Could you check a few things on this model? Use its own coordinates, in mm. A direction names the side the tool comes from. Coordinates: 2 decimals unless noted, no trailing zeros. Order: outer loops, then holes, each group sorted by start corner. A loop starts at its lowest first (then second) coordinate and runs counter-clockwise, first axis right, second up. Notation, with made-up numbers: (72.5, -29) - (123.5, -29) arc R31 cw to (123.5, 6) - close; hole circle Ø2 at (5.5, 34.25). An arc over 180 degrees is marked (long way). Answer as a JSON object with one key per item and string values. Group by question number.
(1) Which directions (+Z, -Z, +X, -X, +Y, -Y) give clear straight access to the entire face, cutting with the end or side of a thin tool? Please do faces 1 (the flat face through (0, -30.5, 2)), 2 (the flat face through (-85, 26, 2)), 3 (the flat face through (1.5, 42, 2)), 4 (the flat face through (-1.5, -42, 2)).
(2) We'd pull the mould along Y, two halves only. Please class faces 5 (the flat face through (-10, 46, 2)), 6 (the flat face through (6, 44.32, 2)), 7 (the flat face through (-85, -26, 2)): pulls with the +Y half, pulls with the -Y half, needs draft (parallel to the pull), parting line crosses it, or undercut.
(3) Please list where these lines run through material, in increasing order: probe 1 along Y at (x, z) = (38.5, 1.35); probe 2 along X at (y, z) = (-42, 1.85); probe 3 along X at (y, z) = (-6, 1.1).
(4) Imagine slicing it at C-C, the plane z = 0.9. Give the number of separate pieces and of enclosed holes in the cut face, and give its area (3 significant figures).
(5) Imagine slicing it at B-B, the plane y = 28.5. Write out the boundary of the cut face in (x, z).
(6) Will these pins go through, and if not, where does the flat tip stop? P1, Ø1.6, axis at y = -46, z = 1, coming from the +X side; P2, Ø1, axis at x = -2.5, z = 1.5, coming from the +Y side; P3, Ø0.6, axis at x = 2.5, z = 1.5, coming from the -Y side.
(7) Imagine slicing it at A-A, the plane x = -17.5. Write out the boundary of the cut face in (y, z), and give its area (3 significant figures).
from build123d import *

# Parameters (mm, degrees)
SKETCH1_W               = 180
SKETCH1_H               = 95
BOSS_EXTRUDE1_DEPTH     = 3.18
CUT_EXTRUDE1_START      = -4.18
SKETCH2_W               = 3.18
SKETCH2_H               = 37.625
CUT_EXTRUDE1_DEPTH      = 5.18
SKETCH3_R               = 1.55
CUT_EXTRUDE2_DEPTH      = 1
CUT_EXTRUDE2_DEPTH_BACK = 4.18
CUT_EXTRUDE3_START      = -4.18
CUT_EXTRUDE3_DEPTH      = 5.18
SKETCH7_W               = 98.6
SKETCH7_H               = 61.9
CUT_EXTRUDE6_DEPTH      = 1
CUT_EXTRUDE6_DEPTH_BACK = 4.18
SKETCH8_W               = 9
SKETCH8_H               = 52
CUT_EXTRUDE7_DEPTH      = 1
CUT_EXTRUDE7_DEPTH_BACK = 4.18


with BuildPart() as part:
    # Sketch1 → Boss-Extrude1 (new body)
    with BuildSketch(Plane.XY):
        Rectangle(SKETCH1_W, SKETCH1_H)
    extrude(amount=BOSS_EXTRUDE1_DEPTH)

    # Sketch2 → Cut-Extrude1 (cut)
    with BuildSketch(Plane.XY.offset(3.18).offset(CUT_EXTRUDE1_START)):
        with Locations((88.41, 28.6875)):
            Rectangle(SKETCH2_W, SKETCH2_H)
    cut_extrude1 = extrude(amount=CUT_EXTRUDE1_DEPTH, mode=Mode.SUBTRACT)

    # Mirror1: Cut-Extrude1 across plane
    add(cut_extrude1.mirror(Plane.ZX), mode=Mode.SUBTRACT)

    # Sketch3 → Cut-Extrude2 (cut, two sides)
    with BuildSketch(Plane.XY.offset(3.18)) as cut_extrude2_sk:
        with Locations((88, -0.125)):
            Circle(SKETCH3_R)
    extrude(amount=CUT_EXTRUDE2_DEPTH, mode=Mode.SUBTRACT)
    extrude(cut_extrude2_sk.sketch, amount=-CUT_EXTRUDE2_DEPTH_BACK, mode=Mode.SUBTRACT)

    # Sketch4 → Cut-Extrude3 (cut)
    with BuildSketch(Plane.XY.offset(3.18).offset(CUT_EXTRUDE3_START)):
        Polygon((-10, -47.5), (10, -47.5), (10, -44.32), (1.5, -44.32), (1.5, -40.318812073), (3.5, -40.318812073), (3.5, -37.5), (1.5, -37.5), (1.5, -34.5), (-1.5, -34.5), (-1.5, -37.5), (-3.5, -37.5), (-3.5, -40.318812073), (-1.5, -40.318812073), (-1.5, -44.32), (-10, -44.32), align=None)
    cut_extrude3 = extrude(amount=CUT_EXTRUDE3_DEPTH, mode=Mode.SUBTRACT)

    # Mirror2: Cut-Extrude3 across plane
    add(cut_extrude3.mirror(Plane.ZX), mode=Mode.SUBTRACT)

    # Sketch7 → Cut-Extrude6 (cut, two sides)
    with BuildSketch(Plane(origin=(0, 0, 0), x_dir=(-1, 0, 0), z_dir=(0, 0, -1))) as cut_extrude6_sk:
        with Locations((0.7, 0.45)):
            Rectangle(SKETCH7_W, SKETCH7_H)
    extrude(amount=CUT_EXTRUDE6_DEPTH, mode=Mode.SUBTRACT)
    extrude(cut_extrude6_sk.sketch, amount=-CUT_EXTRUDE6_DEPTH_BACK, mode=Mode.SUBTRACT)

    # Sketch8 → Cut-Extrude7 (cut, two sides)
    with BuildSketch(Plane(origin=(0, 0, 0), x_dir=(-1, 0, 0), z_dir=(0, 0, -1))) as cut_extrude7_sk:
        with Locations((85.5, 0)):
            Rectangle(SKETCH8_W, SKETCH8_H)
    extrude(amount=CUT_EXTRUDE7_DEPTH, mode=Mode.SUBTRACT)
    extrude(cut_extrude7_sk.sketch, amount=-CUT_EXTRUDE7_DEPTH_BACK, mode=Mode.SUBTRACT)


solid = part.part
Result set:
{
 "1": {"face 1": "+Z, -Z", "face 2": "+Z, -Z, -X", "face 3": "+Z, -Z, +Y", "face 4": "+Z, -Z, -Y"},
 "2": {"face 5": "needs draft", "face 6": "pulls with the +Y half", "face 7": "undercut"},
 "3": {"probe 1": "y = -47.5 to -30.5, 31.4 to 47.5", "probe 2": "x = -90 to -1.5, 1.5 to 86.82", "probe 3": "x = -81 to -50, 48.6 to 90"},
 "4": {"separate pieces": "1", "enclosed holes": "2", "area": "10,100 mm^2"},
 "5": {"outline": "(-90, 0) - (-50, 0) - (-50, 3.18) - (-90, 3.18) - close; (48.6, 0) - (86.82, 0) - (86.82, 3.18) - (48.6, 3.18) - close"},
 "6": {"P1": "stops at x = 86.82", "P2": "stops at y = 44.32", "P3": "stops at y = -44.32"},
 "7": {"outline": "(-47.5, 0) - (-30.5, 0) - (-30.5, 3.18) - (-47.5, 3.18) - close; (31.4, 0) - (47.5, 0) - (47.5, 3.18) - (31.4, 3.18) - close", "area": "105 mm^2"}
}
